Read the model definition and answer for the solid it produces. Units are mm, in the model's axes. Face numbers are marked on the shaded views. A direction names the side the tool comes from. Round coordinates to 2 decimals unless told otherwise and drop trailing zeros. Order: outer loops, then holes, each group sorted by start corner. A loop starts at its lowest first (then second) coordinate and runs counter-clockwise, first axis right, second up.
from build123d import *

# Parameters (mm, degrees)
SKETCH1_R           = 13
BOSS_EXTRUDE1_DEPTH = 45
SKETCH2_R           = 15.225
BOSS_EXTRUDE2_DEPTH = 3.4
SKETCH3_R           = 15.225
BOSS_EXTRUDE3_DEPTH = 1.75
BOSS_EXTRUDE3_TAPER = 45
SKETCH4_W           = 1
SKETCH4_H           = 6
CUT_EXTRUDE1_DEPTH  = 1


with BuildPart() as part:
    # Sketch1 → Boss-Extrude1 (new body)
    with BuildSketch(Plane.XY):
        Circle(SKETCH1_R)
    extrude(amount=-BOSS_EXTRUDE1_DEPTH)

    # Sketch2 → Boss-Extrude2 (add)
    with BuildSketch(Plane.XY):
        Circle(SKETCH2_R)
    extrude(amount=BOSS_EXTRUDE2_DEPTH)

    # Sketch3 → Boss-Extrude3 (add)
    with BuildSketch(Plane.XY.offset(3.4)):
        Circle(SKETCH3_R)
    extrude(amount=BOSS_EXTRUDE3_DEPTH, taper=BOSS_EXTRUDE3_TAPER)

    # Sketch4 → Cut-Extrude1 (cut)
    with BuildSketch(Plane.XY.offset(5.15)):
        Rectangle(SKETCH4_W, SKETCH4_H)
    extrude(amount=-CUT_EXTRUDE1_DEPTH, mode=Mode.SUBTRACT)


solid = part.part
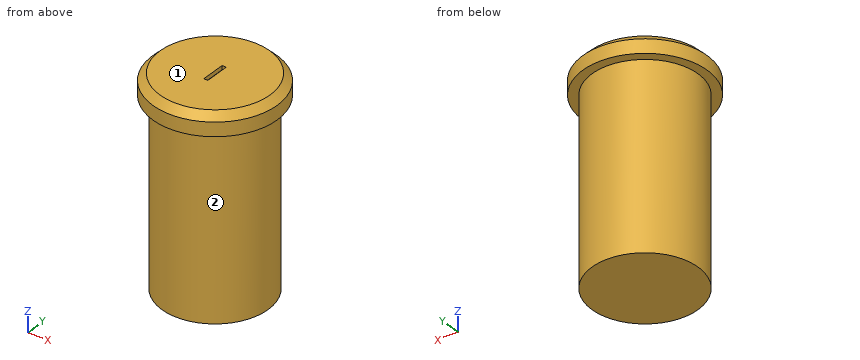
Q1. A cutting plane is placed at B-B, the plane z = -39. Give the vertices of the cut face in (x, y).
Outcome:
outline: circle Ø26 at (0, 0)
Q2. A cutting plane is placed at A-A, the plane y = 0. Give the vertices of the cut face in (x, z) (3 decimals).
Outcome:
outline: (-15.225, 0) - (-13, 0) - (-13, -45) - (13, -45) - (13, 0) - (15.225, 0) - (15.225, 3.4) - (13.475, 5.15) - (0.5, 5.15) - (0.5, 4.15) - (-0.5, 4.15) - (-0.5, 5.15) - (-13.475, 5.15) - (-15.225, 3.4) - close
Q3. Flat-ended cylindrical pins translate along their axes: pin 1 (12 mm diameter, centred on x = -7, z = -27.5, fed in from +Y); pin 2 (2 mm diameter, centred on y = -0.5, z = -23.5, fed in from -X); pin 3 (2 mm diameter, centred on y = -8, z = -31.5, fed in from -X). Find the tip coordinate at first contact, or state that the pin passes through.
Outcome:
pin 1: stops at y = 12.96
pin 2: stops at x = -13
pin 3: stops at x = -10.95
Q4. For the marked faces 1 and 2, determine the directions among +Z, -Z, +X, -X, +Y, -Y from which every point of the face is accessible in a straight line to the end or side of a thin tool.
Outcome:
face 1: +Z, +X, -X, +Y, -Y
face 2: -Z
Q5. Straight lines are drawn through the part: probe 1 along Y at (x, z) = (0, -23); probe 2 along Y at (x, z) = (-1.5, 2); probe 3 along X at (y, z) = (-3.5, -21.5). For each, find the intervals that lie inside material, in ascending order.
Outcome:
probe 1: y = -13 to 13
probe 2: y = -15.15 to 15.15
probe 3: x = -12.52 to 12.52
